Geometry: final body of the model. Coordinates: model frame, mm. A direction names the side the tool comes from. Give positions to 0.01 mm unless a question says otherwise; leave off trailing zeros. Write each loop counter-clockwise with the first axis right and the second up, starting at its lowest first coordinate (ties: lowest second). Pieces come first, ordered by that corner, then holes.
Q1. Line query: line 1 (Z direction, x = 0, y = -1.4) (3 decimals); line 2 (X direction, y = -7, z = 3.5); line 3 (Y direction, x = -6.25, z = 1.75). Output: solid intervals per line, ascending.
Q2. Reachability of faces 4 (the flat face through (6.203, -14.463, -0.1)), 5 (the flat face through (-7.523, -24.5, -1.7)), 6 (the flat face through (4.823, -24, -2)) from +Z, -Z, +X, -X, +Y, -Y: full face, straight path, thin tool, end or side. Return the list, or none.
Q3. Section C-C (x = 0). Return the cut outline in (y, z) (3 decimals).
Q4. Section B-B (x = -5.5). Return the cut outline in (y, z) (3 decimals), plus the area to 3 significant figures.
Q5. Pin query (flat end, axial travel): pin 1 Ø5.5 at (y, z) = (-27.3, 0) entering from -X; pin 2 Ø4.5 at (y, z) = (-24.5, -3) entering from -X; pin 3 Ø4.5 at (x, z) = (-3.5, 2.5) entering from -Y. Return the tip coordinate at first contact, or that it passes through.
Q6. Section A-A (y = -5.5). Return the cut outline in (x, z) (3 decimals), plus the area to 4 significant figures.
Q7. Section D-D (z = 0). State how many separate pieces and enclosed holes the cut face has, plus the area to 3 significant figures.
Q8. Mould query, pull axis X, two halves, no side actions, for faces 1 (the flat face through (7.523, -24.5, -1.7)), 2 (the cylindrical face through (6.15, -34.42, -0.16)), 3 (the flat face through (-4.823, -24, -2)). Classes: +X half, -X half, draft (parallel to the pull), parting line (faces both ways), or undercut.
from build123d import *

# Parameters (mm, degrees)
ESBO_O1_W                      = 20
ESBO_O1_H                      = 14.25
FLANGE_BASE2_DEPTH             = 2.7
ARESTA_FLANGE1_STRIP_W         = 11
ARESTA_FLANGE1_STRIP_H         = 2.7
ARESTA_FLANGE1_STRIP_CUT_DEPTH = 14.25
ARESTA_FLANGE1_DEPTH           = 14.25
ARESTA_FLANGE4_START           = -7.125
ARESTA_FLANGE4_DEPTH           = 14.25
ARESTA_FLANGE4_2_DEPTH         = 14.25
ARESTA_FLANGE5_START           = -7.125
ARESTA_FLANGE5_DEPTH           = 14.25
ARESTA_FLANGE5_2_DEPTH         = 14.25
FILETE1_RADIUS                 = 7.125
FILETE1_LENGTH                 = 2.7
FILETE1_OF_ESPELHAR1_2_RADIUS  = 7.125
FILETE1_OF_ESPELHAR1_2_LENGTH  = 2.7
FURO_DE_DI_METRO_6_1_6_1_1_D   = 6.1
FURO_DE_DI_METRO_9_1_9_1_2_D   = 9.1


# Read off the part's stored shape, not the designer's step: Aresta-Flange4, Aresta-Flange5
# Sheet-metal steps are written as plain solids
with BuildPart() as part:
    # Esboço1 → Flange-base2 (new body)
    with BuildSketch(Plane(origin=(0, 0, 0), x_dir=(1, 0, 0), z_dir=(0, 1, 0))):
        Rectangle(ESBO_O1_W, ESBO_O1_H)
    extrude(amount=-FLANGE_BASE2_DEPTH)

    # Aresta-Flange1 strip (across the edge) → Aresta-Flange1 strip cut (cut)
    with BuildSketch(Plane(origin=(10, -2.7, -7.125), x_dir=(-1, 0, 0), z_dir=(0, 0, 1))):
        with Locations((-2.7, -1.35)):
            Rectangle(ARESTA_FLANGE1_STRIP_W, ARESTA_FLANGE1_STRIP_H)
    aresta_flange1_strip_cut = extrude(amount=ARESTA_FLANGE1_STRIP_CUT_DEPTH, mode=Mode.SUBTRACT)

    # Aresta-Flange1 section (across the edge) → Aresta-Flange1 (add)
    with BuildSketch(Plane(origin=(10, -2.7, -7.125), x_dir=(-1, 0, 0), z_dir=(0, 0, 1))):
        with BuildLine():
            Line((0, 0.1), (0, 15.8))
            Line((0, 15.8), (2.7, 15.8))
            Line((2.7, 15.8), (2.7, 0.1))
            ThreePointArc((2.7, 0.1), (2.729289322, 0.029289322), (2.8, 0))
            Line((2.8, 0), (2.8, -2.7))
            ThreePointArc((2.8, -2.7), (0.820101013, -1.879898987), (0, 0.1))
        make_face()
    aresta_flange1 = extrude(amount=ARESTA_FLANGE1_DEPTH)

    # Aresta-Flange4 outline → Aresta-Flange4 (cut)
    with BuildSketch(Plane.XY.offset(ARESTA_FLANGE4_START)):
        with BuildLine():
            ThreePointArc((10, -12.089086259), (9.93362882, -12.695117178), (9.737661804, -13.272417392))
            Line((9.737661804, -13.272417392), (7.3, -18.5))
            Line((7.3, -18.5), (10, -18.5))
            Line((10, -18.5), (10, -12.089086259))
        make_face()
    aresta_flange4 = extrude(amount=ARESTA_FLANGE4_DEPTH, mode=Mode.SUBTRACT)

    # Aresta-Flange4 2 outline → Aresta-Flange4 2 (add)
    with BuildSketch(Plane.XY.offset(ARESTA_FLANGE4_START)):
        with BuildLine():
            Line((4.822926294, -23.812101706), (7.3, -18.5))
            Line((7.3, -18.5), (7.3, -12.089086259))
            ThreePointArc((7.3, -12.089086259), (7.297629601, -12.11073022), (7.290630779, -12.131348085))
            Line((7.290630779, -12.131348085), (2.375895269, -22.671032399))
            Line((2.375895269, -22.671032399), (4.822926294, -23.812101706))
        make_face()
    aresta_flange4_2 = extrude(amount=ARESTA_FLANGE4_2_DEPTH)

    # Aresta-Flange5 outline → Aresta-Flange5 (cut)
    with BuildSketch(Plane.XY.offset(ARESTA_FLANGE5_START)):
        with BuildLine():
            Line((4.822926294, -23.812101706), (4.822926294, -18.044102487))
            ThreePointArc((4.822926294, -18.044102487), (4.889297474, -17.438071568), (5.08526449, -16.860771354))
            Line((5.08526449, -16.860771354), (2.375895269, -22.671032399))
            Line((2.375895269, -22.671032399), (4.822926294, -23.812101706))
        make_face()
    aresta_flange5 = extrude(amount=ARESTA_FLANGE5_DEPTH, mode=Mode.SUBTRACT)

    # Aresta-Flange5 2 outline → Aresta-Flange5 2 (add)
    with BuildSketch(Plane.XY.offset(ARESTA_FLANGE5_START)):
        with BuildLine():
            Line((7.532295515, -18.001840661), (4.822926294, -23.812101706))
            Line((4.822926294, -23.812101706), (4.822926294, -34.423357431))
            Line((4.822926294, -34.423357431), (7.522926294, -34.423357431))
            Line((7.522926294, -34.423357431), (7.522926294, -18.044102487))
            ThreePointArc((7.522926294, -18.044102487), (7.525296693, -18.022458526), (7.532295515, -18.001840661))
        make_face()
    aresta_flange5_2 = extrude(amount=ARESTA_FLANGE5_2_DEPTH)

    # Filete1: full round fillet: the end face becomes a half cylinder, R = half its width
    filete1_face = Plane((6.172926294, -34.423357431, 0), x_dir=(-1, 0, 0), z_dir=(0, -1, 0))  # on the end face: x along it, z out of the body
    filete1_slab = filete1_face.offset(-FILETE1_RADIUS / 2) * Box(FILETE1_LENGTH, 2 * FILETE1_RADIUS, FILETE1_RADIUS, mode=Mode.PRIVATE)  # the body's end, R deep
    filete1_round = Plane((6.172926294, -27.298357431, 0), x_dir=(0, -1, 0), z_dir=(-1, 0, 0)) * Cylinder(FILETE1_RADIUS, FILETE1_LENGTH, mode=Mode.PRIVATE)  # its axis R under the face
    add(filete1_slab - filete1_round, mode=Mode.SUBTRACT)

    # Espelhar1: Aresta-Flange1 strip cut, Aresta-Flange1, Aresta-Flange4, Aresta-Flange4 2, Aresta-Flange5, Aresta-Flange5 2 across plane
    add(aresta_flange1_strip_cut.mirror(Plane(origin=(0, 0, 0), x_dir=(0, 0, 1), z_dir=(1, 0, 0))), mode=Mode.SUBTRACT)
    add(aresta_flange1.mirror(Plane(origin=(0, 0, 0), x_dir=(0, 0, 1), z_dir=(1, 0, 0))))
    add(aresta_flange4.mirror(Plane(origin=(0, 0, 0), x_dir=(0, 0, 1), z_dir=(1, 0, 0))), mode=Mode.SUBTRACT)
    add(aresta_flange4_2.mirror(Plane(origin=(0, 0, 0), x_dir=(0, 0, 1), z_dir=(1, 0, 0))))
    add(aresta_flange5.mirror(Plane(origin=(0, 0, 0), x_dir=(0, 0, 1), z_dir=(1, 0, 0))), mode=Mode.SUBTRACT)
    add(aresta_flange5_2.mirror(Plane(origin=(0, 0, 0), x_dir=(0, 0, 1), z_dir=(1, 0, 0))))

    # Filete1 of Espelhar1 2: full round fillet: the end face becomes a half cylinder, R = half its width
    filete1_of_espelhar1_2_face = Plane((-6.172926294, -34.423357431, 0), x_dir=(1, 0, 0), z_dir=(0, -1, 0))  # on the end face: x along it, z out of the body
    filete1_of_espelhar1_2_slab = filete1_of_espelhar1_2_face.offset(-FILETE1_OF_ESPELHAR1_2_RADIUS / 2) * Box(FILETE1_OF_ESPELHAR1_2_LENGTH, 2 * FILETE1_OF_ESPELHAR1_2_RADIUS, FILETE1_OF_ESPELHAR1_2_RADIUS, mode=Mode.PRIVATE)  # the body's end, R deep
    filete1_of_espelhar1_2_round = Plane((-6.172926294, -27.298357431, 0), x_dir=(0, -1, 0), z_dir=(1, 0, 0)) * Cylinder(FILETE1_OF_ESPELHAR1_2_RADIUS, FILETE1_OF_ESPELHAR1_2_LENGTH, mode=Mode.PRIVATE)  # its axis R under the face
    add(filete1_of_espelhar1_2_slab - filete1_of_espelhar1_2_round, mode=Mode.SUBTRACT)

    # Furo de diâmetro Ø6.1 (6.1)1 (through all)
    with Locations(Plane(origin=(7.522926294, 0, 0), x_dir=(0, 0, -1), z_dir=(1, 0, 0))):
        with Locations((0, -27.298357431)):
            Hole(FURO_DE_DI_METRO_6_1_6_1_1_D / 2)

    # Furo de diâmetro Ø9.1 (9.1)2 (through all)
    with Locations(Plane(origin=(0, 0, 0), x_dir=(1, 0, 0), z_dir=(0, 1, 0))):
        with Locations((0, 0)):
            Hole(FURO_DE_DI_METRO_9_1_9_1_2_D / 2)


solid = part.part
Computed:
1. line 1: z = -7.125 to -4.55, 4.55 to 7.125
1. line 2: x = -10 to -7.3, 7.3 to 10
1. line 3: y = -34.21 to -29.8, -24.8 to -14.36, -2.7 to 0
2. face 4: +Z, -Z
2. face 5: +Z, -Z, -X, -Y
2. face 6: +Z, -Z, -Y
3. outline: (-2.7, -7.125) - (0, -7.125) - (0, -4.55) - (-2.7, -4.55) - close; (-2.7, 4.55) - (0, 4.55) - (0, 7.125) - (-2.7, 7.125) - close
4. outline: (-27.298, -7.125) - (-15.971, -7.125) - (-15.971, 7.125) - (-27.298, 7.125) arc R7.125 ccw to start; (-2.7, -7.125) - (0, -7.125) - (0, 7.125) - (-2.7, 7.125) - close; hole circle Ø6.1 at (-27.298, 0)
4. area: 250 mm2
5. pin 1: passes through
5. pin 2: stops at x = -7.52
5. pin 3: stops at y = -34.39
6. outline: (-10, -7.125) - (-7.3, -7.125) - (-7.3, 7.125) - (-10, 7.125) - close; (7.3, -7.125) - (10, -7.125) - (10, 7.125) - (7.3, 7.125) - close
6. area: 76.95 mm2
7. separate pieces: 4
7. enclosed holes: 0
7. area: 167 mm2
8. face 1: +X half
8. face 2: draft
8. face 3: undercut
